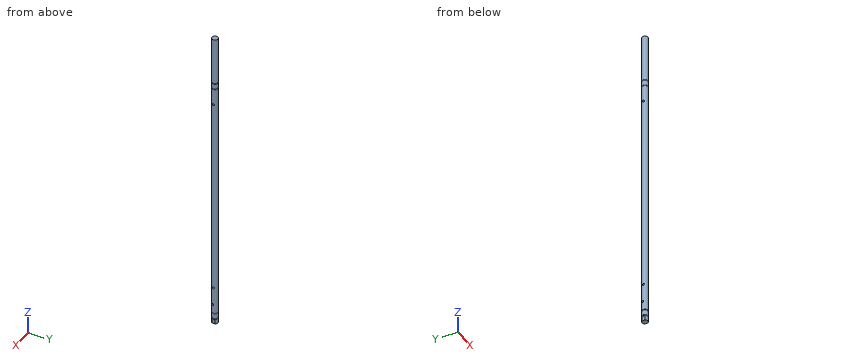
```python
from build123d import *

# Parameters (mm, degrees)
SKETCH1_R                                  = 3
BOSS_EXTRUDE1_DEPTH                        = 275
SKETCH3_W                                  = 0.8
SKETCH3_H                                  = 0.5
CUT_EXTRUDE2_DEPTH                         = 276.032725326
CUT_EXTRUDE2_DEPTH_BACK                    = 276.032725326
SKETCH4_W                                  = 3.470061058
SKETCH4_H                                  = 7
SKETCH4_W_2                                = 2.92528695
CHAMFER1_SIZE                              = 0.3
RETAINING_GROOVES_D5P7_1_START             = 7.05
SKETCH5_R                                  = 2.85
SKETCH5_R_2                                = 2.49
RETAINING_GROOVES_D5P7_1_DEPTH             = 0.8
RETAINING_GROOVES_D5P7_2_START             = 13
SKETCH6_R                                  = 2.85
SKETCH6_R_2                                = 2.49
RETAINING_GROOVES_D5P7_2_DEPTH             = 0.8
RETAINING_GROOVES_D5P7_3_START             = 260.25
SKETCH7_R                                  = 2.85
SKETCH7_R_2                                = 2.49
RETAINING_GROOVES_D5P7_3_DEPTH             = 0.8
RETAINING_GROOVES_D5P7_4_START             = 266.2
SKETCH8_R                                  = 2.85
SKETCH8_R_2                                = 2.49
RETAINING_GROOVES_D5P7_4_DEPTH             = 0.8
TWO_HUB_CROSS_PIN_D2_DEPTH                 = 276.032725326
TWO_HUB_CROSS_PIN_D2_DEPTH_BACK            = 276.032725326
SKETCH9_R                                  = 1
SKETCH10_R                                 = 3.1
REVB_LOWER_SHAFT_NOSE_CLEARANCE_2MM_DEPTH  = 2
REVB_OLDHAM_D2_DRIVE_PIN_CLOCKED_HOLE_OU_W = 1
REVB_OLDHAM_D2_DRIVE_PIN_CLOCKED_HOLE_OU_H = 6.000106441
BENCH_ONEPIECE_SHAFT_END_TO315_START       = 275
SKETCH11_R                                 = 3
BENCH_ONEPIECE_SHAFT_END_TO315_DEPTH       = 40


# Read off the part's stored shape, not the designer's step: RevB_Oldham_D2_Drive_Pin_Clocked_Hole
with BuildPart() as part:
    # Sketch1 → Boss-Extrude1 (new body)
    with BuildSketch(Plane.XY):
        Circle(SKETCH1_R)
    extrude(amount=BOSS_EXTRUDE1_DEPTH)

    # Sketch3 → Cut-Revolve1 (revolve, cut)
    with BuildSketch(Plane(origin=(0, 0, 0), x_dir=(0, 0, -1), z_dir=(1, 0, 0)), mode=Mode.PRIVATE) as cut_revolve1_sk:
        with Locations((-266.6, 2.75)):
            Rectangle(SKETCH3_W, SKETCH3_H)
        with Locations((-260.65, 2.75)):
            Rectangle(SKETCH3_W, SKETCH3_H)
        with Locations((-13.4, 2.75)):
            Rectangle(SKETCH3_W, SKETCH3_H)
        with Locations((-7.45, 2.75)):
            Rectangle(SKETCH3_W, SKETCH3_H)
    revolve(cut_revolve1_sk.sketch.rotate(Axis((0, 0, 263.365004794), (0, 0, -1)), 90), axis=Axis((0, 0, 263.365004794), (0, 0, -1)), mode=Mode.SUBTRACT)

    # Sketch4 → Cut-Extrude2 (cut, two sides: drawn at the far end of the back side and taken through both)
    with BuildSketch(Plane(origin=(0, 0, 0), x_dir=(1, 0, 0), z_dir=(0, 1, 0)).offset(-CUT_EXTRUDE2_DEPTH_BACK)):
        with Locations((4.235030529, -3.5)):
            Rectangle(SKETCH4_W, SKETCH4_H)
        with Locations((-3.962643475, -3.5)):
            Rectangle(SKETCH4_W_2, SKETCH4_H)
    extrude(amount=CUT_EXTRUDE2_DEPTH + CUT_EXTRUDE2_DEPTH_BACK, mode=Mode.SUBTRACT)

    # Chamfer1
    chamfer1_edges = [part.edges().sort_by_distance(p)[0] for p in [
        (0, 3, 0),
        (0, -3, 0),
    ]]
    chamfer(chamfer1_edges, length=CHAMFER1_SIZE)

    # Sketch5 → Retaining_Grooves_D5p7_1 (add)
    with BuildSketch(Plane.XY.offset(RETAINING_GROOVES_D5P7_1_START)):
        Circle(SKETCH5_R)
        Circle(SKETCH5_R_2, mode=Mode.SUBTRACT)
    extrude(amount=RETAINING_GROOVES_D5P7_1_DEPTH)

    # Sketch6 → Retaining_Grooves_D5p7_2 (add)
    with BuildSketch(Plane.XY.offset(RETAINING_GROOVES_D5P7_2_START)):
        Circle(SKETCH6_R)
        Circle(SKETCH6_R_2, mode=Mode.SUBTRACT)
    extrude(amount=RETAINING_GROOVES_D5P7_2_DEPTH)

    # Sketch7 → Retaining_Grooves_D5p7_3 (add)
    with BuildSketch(Plane.XY.offset(RETAINING_GROOVES_D5P7_3_START)):
        Circle(SKETCH7_R)
        Circle(SKETCH7_R_2, mode=Mode.SUBTRACT)
    extrude(amount=RETAINING_GROOVES_D5P7_3_DEPTH)

    # Sketch8 → Retaining_Grooves_D5p7_4 (add)
    with BuildSketch(Plane.XY.offset(RETAINING_GROOVES_D5P7_4_START)):
        Circle(SKETCH8_R)
        Circle(SKETCH8_R_2, mode=Mode.SUBTRACT)
    extrude(amount=RETAINING_GROOVES_D5P7_4_DEPTH)

    # Sketch9 → Two_Hub_Cross_Pin_D2 (cut, two sides: drawn at the far end of the back side and taken through both)
    with BuildSketch(Plane(origin=(0, 0, 0), x_dir=(0, 0, -1), z_dir=(1, 0, 0)).offset(-TWO_HUB_CROSS_PIN_D2_DEPTH_BACK)):
        with Locations((-41.5, 0)):
            Circle(SKETCH9_R)
        with Locations((-243.5, 0)):
            Circle(SKETCH9_R)
    extrude(amount=TWO_HUB_CROSS_PIN_D2_DEPTH + TWO_HUB_CROSS_PIN_D2_DEPTH_BACK, mode=Mode.SUBTRACT)

    # Sketch10 → RevB_Lower_Shaft_Nose_Clearance_2mm (cut)
    with BuildSketch(Plane(origin=(0, 0, 0), x_dir=(-1, 0, 0), z_dir=(0, 0, -1))):
        Circle(SKETCH10_R)
    extrude(amount=-REVB_LOWER_SHAFT_NOSE_CLEARANCE_2MM_DEPTH, mode=Mode.SUBTRACT)

    # RevB_Oldham_D2_Drive_Pin_Clocked_Hole ou → RevB_Oldham_D2_Drive_Pin_Clocked_Hole (revolve, cut)
    with BuildSketch(Plane(origin=(0, 0, 22.925), x_dir=(0.2727065426398811, 0.962097262027807, 0), z_dir=(0, 0, -1))):
        with Locations((0.5, 2.6843e-05)):
            Rectangle(REVB_OLDHAM_D2_DRIVE_PIN_CLOCKED_HOLE_OU_W, REVB_OLDHAM_D2_DRIVE_PIN_CLOCKED_HOLE_OU_H)
    revolve(axis=Axis((0, 0, 22.925), (0.962097262027807, -0.2727065426398811, 0)), mode=Mode.SUBTRACT)

    # Sketch11 → Bench_OnePiece_Shaft_End_To315 (add)
    with BuildSketch(Plane.XY.offset(BENCH_ONEPIECE_SHAFT_END_TO315_START)):
        with Locations(Location((0, 0, 0), (0, 0, 213.557309762))):
            Circle(SKETCH11_R)
    extrude(amount=BENCH_ONEPIECE_SHAFT_END_TO315_DEPTH)


solid = part.part
```
Read the model definition and answer for the solid it produces. Units are mm, in the model's axes. Coordinates: 2 decimals unless noted, no trailing zeros. Loops run counter-clockwise (first coordinate to the right, second up) from the corner with the lowest first, then second, coordinate; pieces in that order, holes last.
(1) Consider line 1 along Z through (x, y) = (-0.25, 0); line 2 along Z through (x, y) = (-1, 0); line 3 along Y through (x, z) = (-0.75, 41.5). Determine where each line is inside the solid, lowest interval first.
Solution:
line 1: z = 2 to 21.93, 23.92 to 40.5, 42.5 to 242.5, 244.5 to 315
line 2: z = 2 to 21.96, 23.89 to 40.5, 42.5 to 242.5, 244.5 to 315
line 3: y = -2.9 to -1, 1 to 2.9
(2) The part is cut by section B-B (x = -1). Count the separate pieces of the cut face and the enclosed holes in it, and give its area (3 significant figures).
Solution:
separate pieces: 1
enclosed holes: 3
area: 1,760 mm2
(3) The part is cut by section A-A (z = 222). Determine the outline of the cut face in (x, y).
Solution:
outline: circle Ø6 at (0, 0)
(4) A flat-ended cylindrical pin translates along its axis: pin 1 Ø1.7 at (y, z) = (0, 4) entering from +X. Find the tip coordinate at first contact, or state that the pin passes through.
Solution:
pin 1: stops at x = 2.5
